For this review, take the finished solid that the model builds, in its own axes (mm). A direction names the side the tool comes from. Round coordinates to 2 decimals unless told otherwise and drop trailing zeros. Order: outer loops, then holes, each group sorted by start corner. A loop starts at its lowest first (then second) coordinate and runs counter-clockwise, first axis right, second up. Notation, with made-up numbers: (-1.5, -23) - (5.5, -23) arc R26 ccw to (5.5, 6) - close; hole circle Ø1 at (29, 33). An arc over 180 degrees is marked (long way). One line per question, with ' | ' between items.
```python
from build123d import *

# Parameters (mm, degrees)
F0_R     = 7.5
F1_DEPTH = 4.5
F2_W     = 4.5
F2_H     = 4.5
F3_DEPTH = 4.5
F4_W     = 37
F4_H     = 5
F5_DEPTH = 4.5


with BuildPart() as f1:
    # F0 (on Top) → F1 (new body)
    with BuildSketch(Plane.XY):
        Polygon((10.5, 21.05), (-10.5, 21.05), (-10.5, -21.05), (-2.25, -21.05), (-2.25, -16.55), (2.25, -16.55), (2.25, -21.05), (10.5, -21.05), align=None)
        Circle(F0_R, mode=Mode.SUBTRACT)
    extrude(amount=F1_DEPTH)

    # F2 (on face) → F3 (join)
    with BuildSketch(Plane(origin=(0, 0, 0), x_dir=(1, 0, 0), z_dir=(0, 0, -1))):
        with Locations((0, -18.8)):
            Rectangle(F2_W, F2_H)
    extrude(amount=F3_DEPTH)

    # F4 (on face) → F5 (join)
    with BuildSketch(Plane.XY.offset(4.5)):
        with Locations((0, 18.55)):
            Rectangle(F4_W, F4_H)
    extrude(amount=-F5_DEPTH)


solid = f1.part
```
(1) Insertion check: pin 1 (1.3 mm diameter, centred on y = -18.5, z = 1.5, fed in from -X); pin 2 (2 mm diameter, centred on y = -19, z = 3, fed in from +X); pin 3 (2 mm diameter, centred on y = 19.5, z = -2.5, fed in from +X). Each pin has a flat end and moves straight along its axis. Give the tip position at first contact, or say it passes through.
Output values:
pin 1: x = -10.5 | pin 2: x = 10.5 | pin 3: x = 2.25
(2) We need section C-C on z = 2.5. State the section outline as (x, y) points, plus the area to 3 significant figures.
Output values:
outline: (-18.5, 16.05) - (-10.5, 16.05) - (-10.5, -21.05) - (-2.25, -21.05) - (-2.25, -16.55) - (2.25, -16.55) - (2.25, -21.05) - (10.5, -21.05) - (10.5, 16.05) - (18.5, 16.05) - (18.5, 21.05) - (-18.5, 21.05) - close; hole circle Ø15 at (0, 0) | area: 767 mm^2
(3) We need section B-B on x = -6. State the section outline as (y, z) points, plus the area to 3 significant figures.
Output values:
outline: (-21.05, 0) - (-4.5, 0) - (-4.5, 4.5) - (-21.05, 4.5) - close; (4.5, 0) - (21.05, 0) - (21.05, 4.5) - (4.5, 4.5) - close | area: 149 mm^2
(4) Mouldability with a two-part tool opening along X and no side actions: class faces 4 (the flat face through (0, 21.05, 2)), 5 (the cylindrical face through (-7.493, 0.33, 2.218)), 6 (the flat face through (2.25, -19, 2)), 7 (the flat face through (2.25, 19, -2)) as released by +X, released by -X, zero draft, split by the parting line, or undercut.
Output values:
face 4: zero draft | face 5: undercut | face 6: undercut | face 7: released by +X
(5) We need section D-D on x = 0. State the section outline as (y, z) points.
Output values:
outline: (-16.55, 0) - (-7.5, 0) - (-7.5, 4.5) - (-16.55, 4.5) - close; (7.5, 0) - (16.55, 0) - (16.55, -4.5) - (21.05, -4.5) - (21.05, 4.5) - (7.5, 4.5) - close
(6) For faces 1 (the flat face through (10.5, -3, 2)), 2 (the flat face through (-2.25, -19, 2)), 3 (the flat face through (-2.25, 19, -2)), list the 3-axis set-ups (+Z, -Z, +X, -X, +Y, -Y) from which the entire face can be reached by the end or side of a thin tool; tool diameter is ignored.
Output values:
face 1: +Z, -Z, +X, -Y | face 2: +Z, -Z, -Y | face 3: -Z, -X, +Y, -Y
(7) For probe 1 along Y at (x, z) = (0, 2.9); probe 2 along X at (y, z) = (-17, 2); probe 3 along Y at (x, z) = (-6, 2.5), list the stretches that pass through material, from the lowest coordinate up. Write a range as [from, to].
Output values:
probe 1: [-16.55, -7.5], [7.5, 21.05] | probe 2: [-10.5, -2.25], [2.25, 10.5] | probe 3: [-21.05, -4.5], [4.5, 21.05]
(8) We need section A-A on y = 0. State the section outline as (x, z) points.
Output values:
outline: (-10.5, 0) - (-7.5, 0) - (-7.5, 4.5) - (-10.5, 4.5) - close; (7.5, 0) - (10.5, 0) - (10.5, 4.5) - (7.5, 4.5) - close
